```python
from build123d import *

# Parameters (mm, degrees)
SKETCH033_W      = 36
SKETCH033_H      = 41
SKETCH033_R      = 1.65
EXTRUDE035_DEPTH = 2
SKETCH039_W      = 14.242
SKETCH039_H      = 2.925
EXTRUDE039_DEPTH = 0.5


with BuildPart() as extrude_displaycase_front:
    # Sketch033 → Extrude035 (new body)
    with BuildSketch(Plane.XY):
        with Locations((13.635, 13)):
            Rectangle(SKETCH033_W, SKETCH033_H)
        with Locations((3, 30.31)):
            Circle(SKETCH033_R, mode=Mode.SUBTRACT)
        with Locations((24.27, 30.31)):
            Circle(SKETCH033_R, mode=Mode.SUBTRACT)
        with Locations((3, -2)):
            Circle(SKETCH033_R, mode=Mode.SUBTRACT)
        with Locations((24.27, -2)):
            Circle(SKETCH033_R, mode=Mode.SUBTRACT)
        Polygon((27.37, 23.21), (27.37, 3.51), (-0.1, 3.51), (-0.1, 23.21), (6.514, 23.21), (6.514, 26.135), (20.756, 26.135), (20.756, 23.21), align=None, mode=Mode.SUBTRACT)
    extrude(amount=-EXTRUDE035_DEPTH)


with BuildPart() as fusion_displaycase_front:
    # Sketch039 → Extrude039 (new body)
    with BuildSketch(Plane.XY):
        with Locations((13.635, 24.6725)):
            Rectangle(SKETCH039_W, SKETCH039_H)
    extrude(amount=-EXTRUDE039_DEPTH)

    # Fusion012: union Extrude_DisplayCase_Front
    add(extrude_displaycase_front.part)


solid = fusion_displaycase_front.part
```
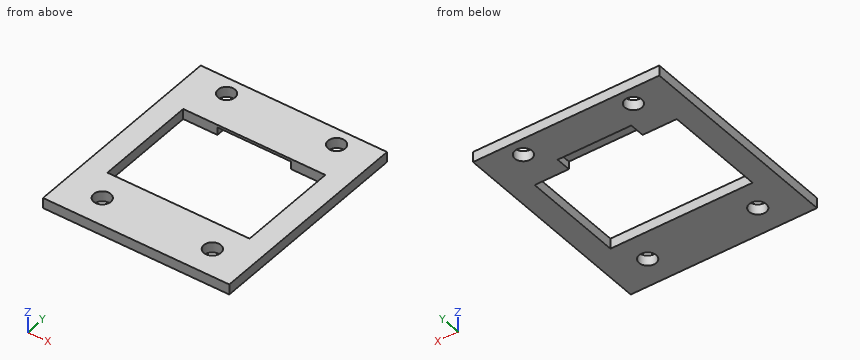
Build history of the part. All positions in model axes, mm. Coordinates: 2 decimals unless noted, no trailing zeros. Write each loop counter-clockwise with the first axis right and the second up, starting at its lowest first coordinate (ties: lowest second). Pieces come first, ordered by that corner, then holes.
1. Band-saw the part on B-B, the plane y = 30.31. Give the cut face in (x, z) (3 decimals).
Answer block:
outline: (-4.365, -2) - (1.35, -2) - (1.35, 0) - (-4.365, 0) - close; (4.65, -2) - (22.62, -2) - (22.62, 0) - (4.65, 0) - close; (25.92, -2) - (31.635, -2) - (31.635, 0) - (25.92, 0) - close
2. Band-saw the part on D-D, the plane y = 9. Give the cut face in (x, z) (3 decimals).
Answer block:
outline: (-4.365, -2) - (-0.1, -2) - (-0.1, 0) - (-4.365, 0) - close; (27.37, -2) - (31.635, -2) - (31.635, 0) - (27.37, 0) - close
3. Band-saw the part on A-A, the plane x = 18. Give the cut face in (y, z) (3 decimals), and give its area (3 significant figures).
Answer block:
outline: (-7.5, -2) - (3.51, -2) - (3.51, 0) - (-7.5, 0) - close; (23.21, -0.5) - (26.135, -0.5) - (26.135, -2) - (33.5, -2) - (33.5, 0) - (23.21, 0) - close
area: 38.2 mm2
4. Band-saw the part on C-C, the plane x = 3. Give the cut face in (y, z), and give its area (3 significant figures).
Answer block:
outline: (-7.5, -2) - (-3.65, -2) - (-3.65, 0) - (-7.5, 0) - close; (-0.35, -2) - (3.51, -2) - (3.51, 0) - (-0.35, 0) - close; (23.21, -2) - (28.66, -2) - (28.66, 0) - (23.21, 0) - close; (31.96, -2) - (33.5, -2) - (33.5, 0) - (31.96, 0) - close
area: 29.4 mm2
5. Drop a flat-ended pin along its axis: pin 1 (1.5 mm diameter, centred on x = 14.5, y = 24.5, fed in from -Z). Give the stop position or say it passes through.
Answer block:
pin 1: stops at z = -0.5
6. Drill centre lines: probe 1 along Y at (x, z) = (3, -0.4); probe 2 along X at (y, z) = (13.5, -0.6) (3 decimals); probe 3 along Y at (x, z) = (9, -1.9) (3 decimals). Where is each one in solid material? Low to high.
Answer block:
probe 1: y = -7.5 to -3.65, -0.35 to 3.51, 23.21 to 28.66, 31.96 to 33.5
probe 2: x = -4.365 to -0.1, 27.37 to 31.635
probe 3: y = -7.5 to 3.51, 26.135 to 33.5
